Design review of the part built by this model. Coordinates are the model's own, in mm. A direction names the side the tool comes from. Round coordinates to 2 decimals unless told otherwise and drop trailing zeros. Loops run counter-clockwise (first coordinate to the right, second up) from the corner with the lowest first, then second, coordinate; pieces in that order, holes last. Notation, with made-up numbers: M -6.75,80 L 16.25,80 A24 ccw 16.25,93 Z; hole C 25.5,19 d3. An arc over 180 degrees is marked long. Use a Markdown table: item, result.
from build123d import *

# Parameters (mm, degrees)
F0_W     = 35
F0_H     = 13
F1_DEPTH = 0.8
F2_W     = 2.4
F2_H     = 2.7
F3_DEPTH = 1.1
F4_R     = 2.5
F5_R     = 0.25
F6_DEPTH = 1.1


# Not quite as in the source:
# - a feature names something its author has since deleted; it is built from what else it names


with BuildPart() as f1:
    # F0 (on Top) → F1 (new body)
    with BuildSketch(Plane.XY):
        Rectangle(F0_W, F0_H)
    extrude(amount=F1_DEPTH)

    # F2 (on face) → F3 (join)
    with BuildSketch(Plane.XY.offset(0.8)):
        with Locations((-12.25, 0)):
            Rectangle(F2_W, F2_H)
        with Locations((-8.75, 0)):
            Rectangle(F2_W, F2_H)
        with Locations((-5.25, 0)):
            Rectangle(F2_W, F2_H)
        with Locations((-1.75, 0)):
            Rectangle(F2_W, F2_H)
        with Locations((1.75, 0)):
            Rectangle(F2_W, F2_H)
        with Locations((5.25, 0)):
            Rectangle(F2_W, F2_H)
        with Locations((8.75, 0)):
            Rectangle(F2_W, F2_H)
        with Locations((12.25, 0)):
            Rectangle(F2_W, F2_H)
    extrude(amount=F3_DEPTH)

    # F4
    f4_edges = [f1.edges().sort_by_distance(p)[0] for p in [
        (-17.5, 6.5, 0.4),
        (-17.5, -6.5, 0.4),
        (17.5, -6.5, 0.4),
        (17.5, 6.5, 0.4),
    ]]
    fillet(f4_edges, radius=F4_R)

    # F5 (on face) → F6 (join)
    with BuildSketch(Plane.XY.offset(0.8)):
        Circle(F5_R)
    extrude(amount=F6_DEPTH)


solid = f1.part
1. Take a section at A-A on z = 1.3. Count the separate pieces of the cut face and the enclosed holes in it, and give its area (3 significant figures).
Check values:
| item | result |
|---|---|
| separate pieces | 9 |
| enclosed holes | 0 |
| area | 52.0 mm² |
2. Wall thickness on line 1 along Z through (x, y) = (3, 4); line 2 along Y through (x, z) = (4.5, 0.9); line 3 along X through (y, z) = (-5.5, 0.55): over which ranges is each line inside the solid? List them lowest first. Write a range as from..to.
Check values:
| item | result |
|---|---|
| line 1 | z = 0..0.8 |
| line 2 | y = -1.35..1.35 |
| line 3 | x = -17..17 |
3. Take a section at B-B on x = 9.5. Give the boundary of the cut face in (y, z), and give its area (3 significant figures).
Check values:
| item | result |
|---|---|
| outline | M -6.5,0 L 6.5,0 L 6.5,0.8 L 1.35,0.8 L 1.35,1.9 L -1.35,1.9 L -1.35,0.8 L -6.5,0.8 Z |
| area | 13.4 mm² |
4. Machinability: for faces 4 (the face through (-12, 1.35, 1)), 5 (the face through (5, -1.35, 1)), 6 (the face through (-2.95, 0, 1)), which of the approach directions +Z, -Z, +X, -X, +Y, -Y give a long, thin tool a straight path to every point of the face, cutting with its end or side? Answer none if there is none.
Check values:
| item | result |
|---|---|
| face 4 | +Z, +X, -X, +Y |
| face 5 | +Z, +X, -X, -Y |
| face 6 | +Z, +Y, -Y |
5. Take a section at C-C on x = -3.5. Give the boundary of the cut face in (y, z).
Check values:
| item | result |
|---|---|
| outline | M -6.5,0 L 6.5,0 L 6.5,0.8 L -6.5,0.8 Z |
6. The part is to be moulded in two halves that separate along X. For faces 1 (the face through (-12, -1.35, 1)), 2 (the face through (6.45, 0, 1)), 3 (the face through (13.45, 0, 1)), say which applies: pulls with the +X half, pulls with the -X half, needs draft (parallel to the pull), parting line crosses it, or undercut.
Check values:
| item | result |
|---|---|
| face 1 | needs draft |
| face 2 | undercut |
| face 3 | pulls with the +X half |
7. Insertion check: pin 1 (1.5 mm diameter, centred on x = 8.5, y = -4, fed in from +Z); pin 2 (0.9 mm diameter, centred on y = 0.5, z = 1.5, fed in from +X); pin 3 (0.9 mm diameter, centred on y = -0.5, z = 1.5, fed in from -X). Each pin has a flat end and moves straight along its axis. Give the tip position at first contact, or say it passes through.
Check values:
| item | result |
|---|---|
| pin 1 | stops at z = 0.8 |
| pin 2 | stops at x = 13.45 |
| pin 3 | stops at x = -13.45 |
